Design review of the part built by this model. Coordinates are the model's own, in mm. A direction names the side the tool comes from. Coordinates: 2 decimals unless noted, no trailing zeros. Loops run counter-clockwise (first coordinate to the right, second up) from the corner with the lowest first, then second, coordinate; pieces in that order, holes last. Notation, with made-up numbers: M 58,63 L 84,63 A15 cw 84,90 Z; hole C -4,74 d11. An arc over 180 degrees is marked long. One line per item, written item: value.
```python
from build123d import *

# Parameters (mm, degrees)
CYLINDER004_R     = 1.25
CYLINDER004_DEPTH = 10
BOX005_W          = 33
BOX005_H          = 2.75
BOX005_DEPTH      = 2
CYLINDER_W        = 4
CYLINDER_H        = 26
CYLINDER_ANGLE    = 180


with BuildPart() as obj1:
    # Cylinder004 → Cylinder004 (new body)
    with BuildSketch(Plane(origin=(10, -1, 4), x_dir=(1, 0, 0), z_dir=(0, 0, 1))):
        Circle(CYLINDER004_R)
    extrude(amount=CYLINDER004_DEPTH)


with BuildPart() as s013:
    # Box005 → Box005 (new body)
    with BuildSketch(Plane(origin=(4, 0, 10), x_dir=(1, 0, 0), z_dir=(0, 0, 1))):
        with Locations((16.5, 1.375)):
            Rectangle(BOX005_W, BOX005_H)
    extrude(amount=BOX005_DEPTH)


with BuildPart() as obj2:
    # Cylinder → Cylinder (revolve)
    with BuildSketch(Plane(origin=(10, 0, -14), x_dir=(-1, 0, 0), z_dir=(0, 1, 0))):
        with Locations((2, 13)):
            Rectangle(CYLINDER_W, CYLINDER_H)
    revolve(axis=Axis((10, 0, -14), (0, 0, 1)), revolution_arc=CYLINDER_ANGLE)

    # Fusion009: union S013
    add(s013.part)

    # Cut015: cut obj1
    add(obj1.part, mode=Mode.SUBTRACT)


with BuildPart() as obj2_1:
    # Cut015 placement: moved
    add(obj2.part.moved(Location((6, 0, 0))))


solid = obj2_1.part
```
(1) We need section A-A on x = 16. State the section outline as (y, z) points, then the cut area to 3 significant figures.
Reply:
outline: M -4,-14 L 0,-14 L 0,4 L -2.25,4 L -2.25,12 L -4,12 Z; M 0.25,10 L 2.75,10 L 2.75,12 L 0.25,12 Z
area: 91.0 mm2
(2) We need section D-D on y = 1.5. State the section outline as (x, z) points.
Reply:
outline: M 10,10 L 43,10 L 43,12 L 10,12 Z
(3) Mouldability with a two-part tool opening along X and no side actions: class faces 4 (the flat face through (31, 0, 11)), 5 (the cylindrical face through (16, -4, -1)), 6 (the flat face through (16, -1, 4)) as released by +X, released by -X, zero draft, split by the parting line, or undercut.
Reply:
face 4: zero draft
face 5: split by the parting line
face 6: undercut
(4) To check wall thickness, follow line 1 along Y through (x, z) = (16, 9.75); line 2 along X through (y, z) = (-1.5, 7.5); line 3 along Z through (x, y) = (18.5, 2.25). State the ranges of each line that lie inside material, in increasing order. Write a range as [from, to].
Reply:
line 1: y = [-4, -2.25]
line 2: x = [12.29, 14.85], [17.15, 19.71]
line 3: z = [10, 12]
(5) We need section B-B on z = -10.75. State the section outline as (x, y) points.
Reply:
outline: M 12,0 A4 ccw 20,0 Z
(6) Insertion check: pin 1 (1.4 mm diameter, centred on x = 33.5, y = 1.5, fed in from -Z); pin 2 (1.5 mm diameter, centred on x = 17, z = -1, fed in from +Y); pin 3 (1.6 mm diameter, centred on x = 31.5, z = 11, fed in from -Y). Each pin has a flat end and moves straight along its axis. Give the tip position at first contact, or say it passes through.
Reply:
pin 1: stops at z = 10
pin 2: stops at y = 0
pin 3: stops at y = 0
(7) Tool access review of faces 1 (the flat face through (26, 1, 10)), 2 (the cylindrical face through (15.73, -2.22, 7.94)), 3 (the flat face through (11, 0, 11)): name each direction out of +Z, -Z, +X, -X, +Y, -Y from which nothing blocks a thin tool from reaching the whole face with its end or side.
Reply:
face 1: -Z, +X, -X, +Y
face 2: +Z
face 3: +Z, -Z, -X, -Y
(8) We need section C-C on x = 29.5. State the section outline as (y, z) points, then the cut area to 3 significant figures.
Reply:
outline: M 0,10 L 2.75,10 L 2.75,12 L 0,12 Z
area: 5.50 mm2
